from build123d import *

# Parameters (mm, degrees)
F1_DEPTH = 25.4
F2_R     = 1.6256
F3_R     = 3.2512


with BuildPart() as f1:
    # F0 (on Front) → F1 (new body)
    with BuildSketch(Plane.XZ):
        Polygon((-1.6256, 0), (0, 0), (0, 19.05), (-19.05, 19.05), (-19.05, 17.4244), (-1.6256, 17.4244), align=None)
    extrude(amount=F1_DEPTH)

    # F2
    f2_edges = [f1.edges().sort_by_distance(p)[0] for p in [
        (-1.6256, -12.7, 17.4244),
    ]]
    fillet(f2_edges, radius=F2_R)

    # F3
    f3_edges = [f1.edges().sort_by_distance(p)[0] for p in [
        (0, -12.7, 19.05),
    ]]
    fillet(f3_edges, radius=F3_R)


solid = f1.part
Check sheet for the modelled part. Datum: model origin and axes. Units: mm. A direction names the side the tool comes from. Coordinates: 2 decimals unless noted, no trailing zeros. Write each loop counter-clockwise with the first axis right and the second up, starting at its lowest first coordinate (ties: lowest second). Pieces come first, ordered by that corner, then holes.
Item 1: Cross-section at B-B on x = -6.5. Record the boundary of the cut face in (y, z).
Numbers:
outline: (-25.4, 17.42) - (0, 17.42) - (0, 19.05) - (-25.4, 19.05) - close
Item 2: Cross-section at A-A on y = -13. Record the boundary of the cut face in (x, z), then the cut area to 3 significant figures.
Numbers:
outline: (-19.05, 17.42) - (-3.25, 17.42) arc R1.63 cw to (-1.63, 15.8) - (-1.63, 0) - (0, 0) - (0, 15.8) arc R3.25 ccw to (-3.25, 19.05) - (-19.05, 19.05) - close
area: 57.6 mm2
Item 3: Access from +Z, -Z, +X, -X, +Y, -Y to the whole of each face (thin tool, end or side, straight path). Record for faces 1 (the face through (-1, -13, 0)), 2 (the face through (-11, -13, 17.424)).
Numbers:
face 1: -Z, +X, -X, +Y, -Y
face 2: -Z, -X, +Y, -Y
Item 4: Cross-section at C-C on z = 9. Record the boundary of the cut face in (x, y).
Numbers:
outline: (-1.63, -25.4) - (0, -25.4) - (0, 0) - (-1.63, 0) - close
Item 5: Scan lines: probe 1 along Z at (x, y) = (-4, -16.25); probe 2 along X at (y, z) = (-14.25, 6.5); probe 3 along X at (y, z) = (-21.5, 18). Record each from-to range of solid material in increasing order.
Numbers:
probe 1: z = 17.42 to 19.05
probe 2: x = -1.63 to 0
probe 3: x = -19.05 to -0.86
Item 6: Depth check by flat-ended pin: pin 1 Ø8 at (y, z) = (-12, 4.5) entering from -X; pin 2 Ø1.5 at (x, y) = (-12.5, -8.5) entering from -Z. Enter the tip coordinate at first touch or a pass-through.
Numbers:
pin 1: stops at x = -1.63
pin 2: stops at z = 17.42
